```python
from build123d import *

# Parameters (mm, degrees)
SKETCH_1_R      = 50
SKETCH_1_R_2    = 25
EXTRUDE_1_DEPTH = 20
SKETCH_2_R      = 25
EXTRUDE_2_DEPTH = 20


with BuildPart() as part:
    # 草图1 → 凸台-拉伸1 (new body)
    with BuildSketch(Plane.XY):
        Circle(SKETCH_1_R)
        with BuildLine():
            Line((302.083333333, 24.913043215), (4.166666667, 49.82608643))
            ThreePointArc((4.166666667, 49.82608643), (36.79900361, 33.850160019), (50, 0))
            ThreePointArc((50, 0), (36.79900361, -33.850160019), (4.166666667, -49.82608643))
            Line((4.166666667, -49.82608643), (302.083333333, -24.913043215))
            ThreePointArc((302.083333333, -24.913043215), (275, 0), (302.083333333, 24.913043215))
        make_face()
        with Locations((300, 0)):
            Circle(SKETCH_1_R_2)
    extrude(amount=EXTRUDE_1_DEPTH)

    # 草图2 → 凸台-拉伸2 (add)
    with BuildSketch(Plane(origin=(0, 0, 0), x_dir=(-1, 0, 0), z_dir=(0, 0, -1))):
        with Locations(Location((0, 0, 0), (0, 0, 180))):
            Circle(SKETCH_2_R)
    extrude(amount=EXTRUDE_2_DEPTH)


solid = part.part
```
Verification items for the finished model (mm, model axes). A direction names the side the tool comes from. Round coordinates to 2 decimals unless told otherwise and drop trailing zeros. Write each loop counter-clockwise with the first axis right and the second up, starting at its lowest first coordinate (ties: lowest second). Pieces come first, ordered by that corner, then holes. Notation, with made-up numbers: (13.25, 16.5) - (35.25, 16.5) arc R28 cw to (35.25, 38.5) - close; hole circle Ø2 at (26, 16.25). An arc over 180 degrees is marked (long way). Answer as a JSON object with one key per item and string values. Group by question number.
Q1. Tool access check on faces 1 (the flat face through (151.04, -37.544, 9.86)), 2 (the cylindrical face through (23.846, -7.509, -9.86)). Record the directions out of +Z, -Z, +X, -X, +Y, -Y that give a thin tool (end or side, any length) a straight path to the whole face; none if there is none.
Q2. Section check D-D, the plane z = 11. Enter the section's corners in (x, y).
Q3. Section check A-A, the plane x = 0. Enter the section's corners in (y, z).
Q4. Thickness scan on line 1 (Y direction, x = -15, z = -12.5); line 2 (Y direction, x = 300.5, z = 14); line 3 (Z direction, x = 9, y = 30.5). Record the ranges inside material, lowest first.
Q5. Section check B-B, the plane y = 0. Enter the section's corners in (x, z), plus the area to 3 significant figures.
Q6. Section check C-C, the plane z = -9. Enter the section's corners in (x, y), plus the area to 3 significant figures.
Q7. Go/stop test with flat-tipped pins: pin 1 Ø1 at (y, z) = (-12.5, 10) entering from +X; pin 2 Ø12 at (y, z) = (10.5, 3.5) entering from +X; pin 3 Ø2 at (x, z) = (1, 7) entering from +Y; pin 4 Ø2 at (x, y) = (218, -33.5) entering from +Z. Record where each tip stops, or that it passes through.
Found:
{
 "1": {"face 1": "+Z, -Z, +X, -Y", "face 2": "-Z"},
 "2": {"outline": "(4.17, -49.83) - (302.08, -24.91) arc R25 ccw to (302.08, 24.91) - (4.17, 49.83) arc R50 ccw (long way) to start"},
 "3": {"outline": "(-50, 0) - (-25, 0) - (-25, -20) - (25, -20) - (25, 0) - (50, 0) - (50, 20) - (-50, 20) - close"},
 "4": {"line 1": "y = -20 to 20", "line 2": "y = -25.05 to 25.05", "line 3": "z = 0 to 20"},
 "5": {"outline": "(-50, 0) - (-25, 0) - (-25, -20) - (25, -20) - (25, 0) - (325, 0) - (325, 20) - (-50, 20) - close", "area": "8,500 mm^2"},
 "6": {"outline": "circle Ø50 at (0, 0)", "area": "1,960 mm^2"},
 "7": {"pin 1": "stops at x = 321.93", "pin 2": "stops at x = 324.59", "pin 3": "stops at y = 50", "pin 4": "passes through"}
}
